from build123d import *

# Parameters (mm, degrees)
SKETCH_1_W          = 12.5
SKETCH_1_H          = 4
EXTRUDE_1_DEPTH     = 4
FILLET_1_R          = 2
SKETCH_1_3_W        = 18.3
SKETCH_1_3_H        = 4
EXTRUDE_2_DEPTH     = 1
FILLET_2_R          = 2
SKETCH_2_R          = 0.75
CUT_EXTRUDE_1_DEPTH = 10.834759784
EXTRUDE_START       = -4
SKETCH_3_R          = 0.5
EXTRUDE_3_DEPTH     = 5.6


with BuildPart() as part:
    # 草图1 → 凸台-拉伸1 (new body)
    with BuildSketch(Plane(origin=(0, 0, 0), x_dir=(1, 0, 0), z_dir=(0, 1, 0))):
        Rectangle(SKETCH_1_W, SKETCH_1_H)
    extrude(amount=EXTRUDE_1_DEPTH)

    # 圆角1
    fillet_1_edges = [part.edges().sort_by_distance(p)[0] for p in [
        (6.25, 2, -2),
        (6.25, 2, 2),
        (-6.25, 2, 2),
        (-6.25, 2, -2),
    ]]
    fillet(fillet_1_edges, radius=FILLET_1_R - 0.0001)  # a hair under: the kernel refuses the full size

    # 草图1<3> → 凸台-拉伸2 (add)
    with BuildSketch(Plane(origin=(0, 0, 0), x_dir=(1, 0, 0), z_dir=(0, 1, 0))):
        Rectangle(SKETCH_1_3_W, SKETCH_1_3_H)
    extrude(amount=EXTRUDE_2_DEPTH)

    # 圆角2
    fillet_2_edges = [part.edges().sort_by_distance(p)[0] for p in [
        (9.15, 0.5, 2),
        (9.15, 0.5, -2),
        (-9.15, 0.5, 2),
        (-9.15, 0.5, -2),
    ]]
    fillet(fillet_2_edges, radius=FILLET_2_R - 0.0001)  # a hair under: the kernel refuses the full size

    # 草图2 → 切除-拉伸1 (cut, through all)
    with BuildSketch(Plane(origin=(0, 1, 0), x_dir=(1, 0, 0), z_dir=(0, 1, 0))):
        with Locations(Location((-7.7, 0, 0), (0, 0, 270))):
            Circle(SKETCH_2_R)
        with Locations(Location((7.7, 0, 0), (0, 0, 270))):
            Circle(SKETCH_2_R)
    extrude(amount=-CUT_EXTRUDE_1_DEPTH, mode=Mode.SUBTRACT)

    # 草图3 → 凸台-拉伸3 (add)
    with BuildSketch(Plane.XZ.offset(EXTRUDE_START)):
        with Locations(Location((-1.27, 0, 0), (0, 0, 90))):
            Circle(SKETCH_3_R)
        with Locations(Location((1.27, 0, 0), (0, 0, 90))):
            Circle(SKETCH_3_R)
    extrude(amount=EXTRUDE_3_DEPTH)


solid = part.part
Source: CAD feature listing. Evaluate the final solid. Frame: model axes, mm. A direction names the side the tool comes from. Round coordinates to 2 decimals unless told otherwise and drop trailing zeros. Loops run counter-clockwise (first coordinate to the right, second up) from the corner with the lowest first, then second, coordinate; pieces in that order, holes last. Notation, with made-up numbers: M -36.5,-32.5 L -9.5,-32.5 A10 cw -9.5,-23.5 Z; hole C 33.25,-1.5 d1. An arc over 180 degrees is marked long. Return JSON: item names as keys, results as strings. Group by question number.
1. Material intervals for line 1 along X through (y, z) = (0.5, 0); line 2 along Y through (x, z) = (-5.75, 0.35); line 3 along Y through (x, z) = (6.25, -1.1), sorted ascending. Write a range as from..to.
2. Section query C-C on x = -7.7. Output: boundary loops of the cut face in (y, z).
3. Reachability of faces 4 (the face through (5.65, 2.52, 1.43)), 5 (the face through (-5.68, 2.52, -1.4)), 6 (the face through (-5.68, 2.52, 1.4)), 7 (the face through (5.68, 2.52, -1.4)) from +Z, -Z, +X, -X, +Y, -Y: full face, straight path, thin tool, end or side. Return the list, or none.
4. Section query A-A on y = 0.5. State how many separate pieces and enclosed holes the cut face has, and give its area (3 significant figures).
5. Section query B-B on z = 0.2. Output: boundary loops of the cut face in (x, y).
6. Mould query, pull axis X, two halves, no side actions, for faces 1 (the face through (8.58, 0.51, -1.4)), 2 (the face through (0.774, -0.789, -0.065)), 3 (the face through (0, 2, -2)). Classes: released by +X, released by -X, zero draft, split by the parting line, or undercut.
7. Pin query (flat end, axial travel): pin 1 (1 mm diameter, centred on x = -0.5, z = 0.5, fed in from -Y); pin 2 (1 mm diameter, centred on y = 3.5, z = 0.5, fed in from +X); pin 3 (1.5 mm diameter, centred on x = 7, z = -0.5, fed in from +Y); pin 4 (0.9 mm diameter, centred on x = -7.7, z = 0, fed in from +Y). Return the tip coordinate at first contact, or that it passes through.
Checks:
{
 "1": {"line 1": "x = -9.15..-8.45, -6.95..6.95, 8.45..9.15", "line 2": "y = 0..4", "line 3": "y = 0..1"},
 "2": {"outline": "M 0,-1.92 L 1,-1.92 L 1,-0.75 L 0,-0.75 Z; M 0,0.75 L 1,0.75 L 1,1.92 L 0,1.92 Z"},
 "3": {"face 4": "+Z, +X, +Y", "face 5": "-Z, -X, +Y", "face 6": "+Z, -X, +Y", "face 7": "-Z, +X, +Y"},
 "4": {"separate pieces": "1", "enclosed holes": "2", "area": "66.2 mm²"},
 "5": {"outline": "M -9.14,0 L -8.42,0 L -8.42,1 L -9.14,1 Z; M -6.98,0 L -1.73,0 L -1.73,-1.6 L -0.81,-1.6 L -0.81,0 L 0.81,0 L 0.81,-1.6 L 1.73,-1.6 L 1.73,0 L 6.98,0 L 6.98,1 L 6.24,1 L 6.24,4 L -6.24,4 L -6.24,1 L -6.98,1 Z; M 8.42,0 L 9.14,0 L 9.14,1 L 8.42,1 Z"},
 "6": {"face 1": "released by +X", "face 2": "undercut", "face 3": "zero draft"},
 "7": {"pin 1": "stops at y = -1.6", "pin 2": "stops at x = 6.25", "pin 3": "stops at y = 1", "pin 4": "passes through"}
}
